from build123d import *

# Parameters (mm, degrees)
F2_R    = 1.5
F3_SIZE = 0.75
F4_R    = 2


with BuildPart() as f1:
    # F0 (on Front) → F1 (revolve)
    with BuildSketch(Plane.XZ):
        Polygon((3.4, 8.050387), (3.4, 8), (4.6, 8), (4.6, 15), (3.4, 15), align=None)
        Polygon((3.4, 6.550387), (5.95, 4.000387), (5.95, 8), (4.6, 8), (3.4, 8), align=None)
        Polygon((5.95, 4.000387), (5.95, 0), (7.95, 0), (7.95, 8), (5.95, 8), align=None)
    revolve(axis=Axis((0, 0, 34.607098), (0, 0, 1)))

    # F2
    f2_edges = [f1.edges().sort_by_distance(p)[0] for p in [
        (-7.95, 0, 8),
        (-7.95, 0, 0),
    ]]
    fillet(f2_edges, radius=F2_R)

    # F3
    f3_edges = [f1.edges().sort_by_distance(p)[0] for p in [
        (-4.6, 0, 15),
    ]]
    chamfer(f3_edges, length=F3_SIZE)

    # F4
    f4_edges = [f1.edges().sort_by_distance(p)[0] for p in [
        (-3.4, 0, 6.550387),
        (-5.95, 0, 4.000387),
    ]]
    fillet(f4_edges, radius=F4_R)


solid = f1.part
Read the model definition and answer for the solid it produces. Units are mm, in the model's axes. A direction names the side the tool comes from. Round coordinates to 2 decimals unless told otherwise and drop trailing zeros. Loops run counter-clockwise (first coordinate to the right, second up) from the corner with the lowest first, then second, coordinate; pieces in that order, holes last.
Q1. Consider probe 1 along X at (y, z) = (0.75, 5.5); probe 2 along Z at (x, y) = (5.5, 2.75); probe 3 along X at (y, z) = (-2.5, 6). Determine where each line is inside the solid, lowest interval first.
Q2. Section A-A on z = 1 is taken. Write down the section's boundary in (x, y).
Q3. Each of these flat-tipped pins is pushed along its axis until it touches: pin 1 (3 mm diameter, centred on x = -2, z = 11, fed in from -Y); pin 2 (8 mm diameter, centred on y = -1.5, z = 13, fed in from +X); pin 3 (1.5 mm diameter, centred on y = -3.5, z = 2.5, fed in from -X). Where does it stop, or does it pass through?
Q4. Which of the six approach directions +Z, -Z, +X, -X, +Y, -Y give full straight-line access (tool end or side, diameter ignored) to faces 1 (the face through (5.496, -2.279, 1.564)), 2 (the face through (2, -3, 15)), 3 (the face through (-3.65, -2.8, 11.17))?
Output:
1. probe 1: x = -7.91 to -4.39, 4.39 to 7.91
1. probe 2: z = 0 to 8
1. probe 3: x = -7.55 to -3.06, 3.06 to 7.55
2. outline: circle Ø15.73 at (0, 0); hole circle Ø11.9 at (0, 0)
3. pin 1: stops at y = -4.57
3. pin 2: stops at x = 4.6
3. pin 3: stops at x = -7.46
4. face 1: -Z
4. face 2: +Z, +X, -X, +Y, -Y
4. face 3: +Z
